Model file for the job. Use its own axes, mm. A direction names the side the tool comes from. Round coordinates to 2 decimals unless told otherwise and drop trailing zeros. Order: outer loops, then holes, each group sorted by start corner. A loop starts at its lowest first (then second) coordinate and runs counter-clockwise, first axis right, second up. Notation, with made-up numbers: M -10.75,25 L -5.75,25 A10 cw -5.75,40 Z; hole C -26.75,58.5 d7. An arc over 180 degrees is marked long. Return JSON: item names as keys, results as strings. Group by question number.
Item 1: Slice it at B-B on y = 3.5. Give the number of separate pieces and of enclosed holes in the cut face, then the cut area to 3 significant figures.
Item 2: Pin check, flat tips, straight feed: pin 1 Ø11.5 at (x, z) = (-9.85, 0) entering from -Y; pin 2 Ø1.1 at (x, z) = (-16.85, 0) entering from +Y; pin 3 Ø10.5 at (x, z) = (-7.5, 4.5) entering from +Y. Stop position of each tip, or through.
Item 3: Slice it at D-D on x = -8. Write the cut outline in (y, z).
Item 4: Pull direction X, two halves, no side cores. Call faces 1 (the face through (-17, 3.8, -13.6)), 2 (the face through (-3.74, 2.45, 0.12)), 3 (the face through (0, 7.46, 5)), 4 (the face through (-30.15, 4, 0)): pulls with the +X half, pulls with the -X half, needs draft (parallel to the pull), parting line crosses it, or undercut.
Item 5: Slice it at A-A on x = -25. Write the cut outline in (y, z).
Item 6: Which spindle directions (+Z, -Z, +X, -X, +Y, -Y) get a long thin tool onto all of the face, cutting with end or side? Do faces 5 (the face through (0, 4, 22.25)), 6 (the face through (-12, 4.96, 5)). Say none if no direction does.
Item 7: Probe line 1 along X through (y, z) = (2.05, 0); line 2 along X through (y, z) = (6.05, 0); line 3 along Z through (x, y) = (-22.5, 6.5). List the from-to ranges inside material, lowest first.
Item 8: Slice it at C-C on z = 0. Write the cut outline in (x, y), then the cut area to 3 significant figures.
from build123d import *

# Parameters (mm, degrees)
SKETCH3_W           = 60.3
SKETCH3_H           = 44.5
SKETCH3_R           = 0.9
SKETCH3_R_2         = 4.9
BOSS_EXTRUDE1_DEPTH = 7.46
SKETCH4_R           = 10.5
CUT_EXTRUDE1_DEPTH  = 2.5
SKETCH5_R           = 2.6
CUT_EXTRUDE2_DEPTH  = 39.206499447


with BuildPart() as part:
    # Sketch3 → Boss-Extrude1 (new body)
    with BuildSketch(Plane(origin=(0, 0, 0), x_dir=(1, 0, 0), z_dir=(0, 1, 0))):
        Rectangle(SKETCH3_W, SKETCH3_H)
        with Locations(Location((-9.85, 7, 0), (0, 0, 90))):
            Circle(SKETCH3_R, mode=Mode.SUBTRACT)
        with Locations(Location((-16.85, 0, 0), (0, 0, 90))):
            Circle(SKETCH3_R, mode=Mode.SUBTRACT)
        with Locations(Location((-9.85, -7, 0), (0, 0, 90))):
            Circle(SKETCH3_R, mode=Mode.SUBTRACT)
        with Locations(Location((-2.85, 0, 0), (0, 0, 90))):
            Circle(SKETCH3_R, mode=Mode.SUBTRACT)
        with Locations(Location((-9.85, 0, 0), (0, 0, 90))):
            Circle(SKETCH3_R_2, mode=Mode.SUBTRACT)
    extrude(amount=BOSS_EXTRUDE1_DEPTH)

    # Sketch4 → Cut-Extrude1 (cut)
    with BuildSketch(Plane(origin=(0, 7.46, 0), x_dir=(1, 0, 0), z_dir=(0, 1, 0))):
        with Locations(Location((-9.85, 0, 0), (0, 0, 270))):
            Circle(SKETCH4_R)
    extrude(amount=-CUT_EXTRUDE1_DEPTH, mode=Mode.SUBTRACT)

    # Sketch5 → Cut-Extrude2 (cut, through all)
    with BuildSketch(Plane(origin=(0, 7.46, 0), x_dir=(1, 0, 0), z_dir=(0, 1, 0))):
        with Locations(Location((0, 16, 0), (0, 0, 270))):
            Circle(SKETCH5_R)
        with Locations(Location((8, 16, 0), (0, 0, 270))):
            Circle(SKETCH5_R)
        with Locations(Location((16, 16, 0), (0, 0, 270))):
            Circle(SKETCH5_R)
        with Locations(Location((24, 16, 0), (0, 0, 270))):
            Circle(SKETCH5_R)
        with Locations(Location((-24, 16, 0), (0, 0, 270))):
            Circle(SKETCH5_R)
        with Locations(Location((-16, 16, 0), (0, 0, 270))):
            Circle(SKETCH5_R)
        with Locations(Location((-8, 16, 0), (0, 0, 270))):
            Circle(SKETCH5_R)
        with Locations(Location((-8, -16, 0), (0, 0, 270))):
            Circle(SKETCH5_R)
        with Locations(Location((-16, -16, 0), (0, 0, 270))):
            Circle(SKETCH5_R)
        with Locations(Location((-24, -16, 0), (0, 0, 270))):
            Circle(SKETCH5_R)
        with Locations(Location((24, -16, 0), (0, 0, 270))):
            Circle(SKETCH5_R)
        with Locations(Location((16, -16, 0), (0, 0, 270))):
            Circle(SKETCH5_R)
        with Locations(Location((8, -16, 0), (0, 0, 270))):
            Circle(SKETCH5_R)
        with Locations(Location((0, -16, 0), (0, 0, 270))):
            Circle(SKETCH5_R)
    extrude(amount=-CUT_EXTRUDE2_DEPTH, mode=Mode.SUBTRACT)


solid = part.part
Output values:
{
 "1": {"separate pieces": "1", "enclosed holes": "19", "area": "2,300 mm²"},
 "2": {"pin 1": "y = 0", "pin 2": "through", "pin 3": "y = 4.96"},
 "3": {"outline": "M 0,-22.25 L 7.46,-22.25 L 7.46,-18.6 L 0,-18.6 Z; M 0,-13.4 L 7.46,-13.4 L 7.46,-10.34 L 4.96,-10.34 L 4.96,-4.54 L 0,-4.54 Z; M 0,4.54 L 4.96,4.54 L 4.96,10.34 L 7.46,10.34 L 7.46,13.4 L 0,13.4 Z; M 0,18.6 L 7.46,18.6 L 7.46,22.25 L 0,22.25 Z"},
 "4": {"face 1": "undercut", "face 2": "undercut", "face 3": "needs draft", "face 4": "pulls with the -X half"},
 "5": {"outline": "M 0,-22.25 L 7.46,-22.25 L 7.46,-18.4 L 0,-18.4 Z; M 0,-13.6 L 7.46,-13.6 L 7.46,13.6 L 0,13.6 Z; M 0,18.4 L 7.46,18.4 L 7.46,22.25 L 0,22.25 Z"},
 "6": {"face 5": "+Z, +X, -X, +Y, -Y", "face 6": "+Y"},
 "7": {"line 1": "-30.15 to -17.75, -15.95 to -14.75, -4.95 to -3.75, -1.95 to 30.15", "line 2": "-30.15 to -20.35, 0.65 to 30.15", "line 3": "-22.25 to -18.12, -13.88 to 13.88, 18.12 to 22.25"},
 "8": {"outline": "M -30.15,0 L -17.75,0 L -17.75,4.96 L -20.35,4.96 L -20.35,7.46 L -30.15,7.46 Z; M -15.95,0 L -14.75,0 L -14.75,4.96 L -15.95,4.96 Z; M -4.95,0 L -3.75,0 L -3.75,4.96 L -4.95,4.96 Z; M -1.95,0 L 30.15,0 L 30.15,7.46 L 0.65,7.46 L 0.65,4.96 L -1.95,4.96 Z", "area": "331 mm²"}
}
